Can you work these out from the model? Positions are in its coordinate system, mm. Coordinates: 2 decimals unless noted, no trailing zeros. Use one line per item in the form item = value. Start each with the question number.
(1) I'm going to push flat-ended pins straight in: pin 1 (2 mm diameter, centred on y = 16.5, z = 5.5, fed in from -X); pin 2 (2.5 mm diameter, centred on y = -16.5, z = 7, fed in from +X); pin 3 (2.5 mm diameter, centred on x = 0, y = 8, fed in from +Z); pin 4 (3 mm diameter, centred on y = -16.5, z = 6.5, fed in from +X). Where does each tip first touch, or does it pass through?
(2) I need wall thicknesses on line 1 (Y direction, x = 0, z = 6); line 2 (Y direction, x = -4.5, z = 4.5); line 3 (Y direction, x = -8, z = 7.25). Which ranges of each line are inside material? Lowest first, please. Write a range as [from, to].
(3) Imagine slicing it at A-A (x = 14.5). State how many separate pieces and enclosed holes the cut face has, plus the area to 3 significant figures.
```python
from build123d import *

# Parameters (mm, degrees)
SKETCH_1_R                  = 27.5
EXTRUDE_1_DEPTH             = 10
CUT_EXTRUDE_1_REACH         = 42.156
SKETCH_2_R                  = 22.5
SKETCH_3_R                  = 12.5
EXTRUDE_2_DEPTH             = 10
EXTRUDE_START               = 10
EXTRUDE_3_DEPTH             = 10
HOLE_WIZARD_M32_D           = 3.4
HOLE_WIZARD_M32_CSINK_D     = 3.45
HOLE_WIZARD_M32_CSINK_ANGLE = 90
FILLET_1_R                  = 1


with BuildPart() as part:
    # Sketch 1 → Extrude 1 (new body)
    with BuildSketch(Plane.XY):
        Circle(SKETCH_1_R)
    extrude(amount=EXTRUDE_1_DEPTH)

    # Sketch 2 → Cut-Extrude 1 (cut, up to next)
    with BuildSketch(Plane.XY.offset(10), mode=Mode.PRIVATE) as cut_extrude_1_sk1:
        Circle(SKETCH_2_R)
    cut_extrude_1_tool1 = extrude(cut_extrude_1_sk1.sketch, amount=-CUT_EXTRUDE_1_REACH, mode=Mode.PRIVATE) & part.part
    add(cut_extrude_1_tool1.solids().sort_by_distance((0, 0, 10))[0], mode=Mode.SUBTRACT)



with BuildPart() as body_2:
    # Sketch 3 → Extrude 2 (new body)
    with BuildSketch(Plane.XY):
        Circle(SKETCH_3_R)
    extrude(amount=EXTRUDE_2_DEPTH)


with BuildPart() as part_1:
    add(part.part)

    add(body_2.part)  # Extrude 3 merges body 2
    # Sketch 5 → Extrude 3 (add)
    with BuildSketch(Plane.XY.offset(EXTRUDE_START)):
        with BuildLine():
            Line((9.356601718, 8.288787866), (18.114916731, 13.345403397))
            ThreePointArc((18.114916731, 13.345403397), (19.485571585, 11.25), (20.614916731, 9.015276378))
            Line((20.614916731, 9.015276378), (11.856601718, 3.958660847))
            ThreePointArc((11.856601718, 3.958660847), (10.825317547, 6.25), (9.356601718, 8.288787866))
        make_face()
        with BuildLine():
            Line((2.5, 12.247448714), (2.5, 22.360679775))
            ThreePointArc((2.5, 22.360679775), (0, 22.5), (-2.5, 22.360679775))
            Line((-2.5, 22.360679775), (-2.5, 12.247448714))
            ThreePointArc((-2.5, 12.247448714), (0, 12.5), (2.5, 12.247448714))
        make_face()
        with BuildLine():
            Line((11.856601718, -3.958660847), (20.614916731, -9.015276378))
            ThreePointArc((20.614916731, -9.015276378), (19.485571585, -11.25), (18.114916731, -13.345403397))
            Line((18.114916731, -13.345403397), (9.356601718, -8.288787866))
            ThreePointArc((9.356601718, -8.288787866), (10.825317547, -6.25), (11.856601718, -3.958660847))
        make_face()
        with BuildLine():
            Line((2.5, -12.247448714), (2.5, -22.360679775))
            ThreePointArc((2.5, -22.360679775), (0, -22.5), (-2.5, -22.360679775))
            Line((-2.5, -22.360679775), (-2.5, -12.247448714))
            ThreePointArc((-2.5, -12.247448714), (0, -12.5), (2.5, -12.247448714))
        make_face()
        with BuildLine():
            Line((-9.356601718, -8.288787866), (-18.114916731, -13.345403397))
            ThreePointArc((-18.114916731, -13.345403397), (-19.485571585, -11.25), (-20.614916731, -9.015276378))
            Line((-20.614916731, -9.015276378), (-11.856601718, -3.958660847))
            ThreePointArc((-11.856601718, -3.958660847), (-10.825317547, -6.25), (-9.356601718, -8.288787866))
        make_face()
        with BuildLine():
            Line((-11.856601718, 3.958660847), (-20.614916731, 9.015276378))
            ThreePointArc((-20.614916731, 9.015276378), (-19.485571585, 11.25), (-18.114916731, 13.345403397))
            Line((-18.114916731, 13.345403397), (-9.356601718, 8.288787866))
            ThreePointArc((-9.356601718, 8.288787866), (-10.825317547, 6.25), (-11.856601718, 3.958660847))
        make_face()
    extrude(amount=-EXTRUDE_3_DEPTH)

    # Hole Wizard M32 (through all)
    with Locations(Plane.XY.offset(10)):
        with Locations((-8, 0), (0, 8), (8.225054206, 0), (0, -8)):
            CounterSinkHole(HOLE_WIZARD_M32_D / 2, HOLE_WIZARD_M32_CSINK_D / 2, counter_sink_angle=HOLE_WIZARD_M32_CSINK_ANGLE)

    # Fillet 1
    fillet_1_edges = [part_1.edges().sort_by_distance(p)[0] for p in [
        (-2.5, 12.247448714, 5),
        (2.5, 12.247448714, 5),
        (2.5, 22.360679775, 5),
        (-2.5, 22.360679775, 5),
        (9.356601718, 8.288787866, 5),
        (11.856601718, 3.958660847, 5),
        (20.614916731, 9.015276378, 5),
        (18.114916731, 13.345403397, 5),
        (11.856601718, -3.958660847, 5),
        (9.356601718, -8.288787866, 5),
        (18.114916731, -13.345403397, 5),
        (20.614916731, -9.015276378, 5),
        (2.5, -12.247448714, 5),
        (-2.5, -12.247448714, 5),
        (-2.5, -22.360679775, 5),
        (2.5, -22.360679775, 5),
        (-9.356601718, -8.288787866, 5),
        (-11.856601718, -3.958660847, 5),
        (-20.614916731, -9.015276378, 5),
        (-18.114916731, -13.345403397, 5),
        (-11.856601718, 3.958660847, 5),
        (-9.356601718, 8.288787866, 5),
        (-18.114916731, 13.345403397, 5),
        (-20.614916731, 9.015276378, 5),
    ]]
    fillet(fillet_1_edges, radius=FILLET_1_R)

    # Sweep 2: sweep along a curve in space
    with BuildLine() as sweep_2_path:
        ThreePointArc((27.5, 0, 10), (19.445436483, 19.445436483, 10), (0, 27.5, 10))
        ThreePointArc((0, 27.5, 10), (-19.445436483, 19.445436483, 10), (-27.5, 0, 10))
        ThreePointArc((-27.5, 0, 10), (-19.445436483, -19.445436483, 10), (0, -27.5, 10))
        ThreePointArc((0, -27.5, 10), (19.445436483, -19.445436483, 10), (27.5, 0, 10))
    # Sketch 13 → Sweep 2 (sweep, cut)
    with BuildSketch(Plane(origin=(0, 0, 0), x_dir=(0, 0, -1), z_dir=(1, 0, 0))):
        Polygon((-8, 25.5), (-2, 25.5), (-1, 27.5), (-9, 27.5), align=None)
    sweep(path=sweep_2_path.line, mode=Mode.SUBTRACT)


solid = part_1.part
```
Worked out:
q1.pin_1 = -20.25
q1.pin_2 = 20.44
q1.pin_3 = through
q1.pin_4 = 20.62
q2.line_1 = [-25.5, -9.7], [-6.3, 6.3], [9.7, 25.5]
q2.line_2 = [-25.1, -22.05], [-11.66, 11.66], [22.05, 25.1]
q2.line_3 = [-24.21, -21.03], [-9.6, -1.7], [1.7, 9.6], [21.03, 24.21]
q3.separate_pieces = 4
q3.enclosed_holes = 0
q3.area = 205 mm2
